Work out the finished part from the listing and answer in its coordinate system (mm). A direction names the side the tool comes from. Give positions to 0.01 mm unless a question says otherwise; leave off trailing zeros. Loops run counter-clockwise (first coordinate to the right, second up) from the corner with the lowest first, then second, coordinate; pieces in that order, holes last.
```python
from build123d import *

# Parameters (mm, degrees)
SKETCH_1_W          = 80.1
SKETCH_1_H          = 60.1
EXTRUDE_1_DEPTH     = 28
CUT_EXTRUDE_1_DEPTH = 108
CUT_EXTRUDE_2_DEPTH = 80
FILLET_1_R          = 2
SKETCH_4_R          = 1.8
CUT_EXTRUDE_3_DEPTH = 80
FILLET_2_R          = 10
FILLET_3_R          = 2


with BuildPart() as part:
    # 草图1 → 凸台-拉伸1 (new body)
    with BuildSketch(Plane.XY):
        with Locations((40.05, -30.05)):
            Rectangle(SKETCH_1_W, SKETCH_1_H)
    extrude(amount=EXTRUDE_1_DEPTH)

    # 草图2 → 切除-拉伸1 (cut)
    with BuildSketch(Plane(origin=(80.1, 0, 0), x_dir=(0, 0, -1), z_dir=(1, 0, 0))):
        with BuildLine():
            ThreePointArc((-4, -32), (-6.928932188, -24.928932188), (-14, -22))
            Line((-14, -22), (-14, -32))
            Line((-14, -32), (-4, -32))
        make_face()
        with BuildLine():
            Line((-14, -32), (-14, -22))
            ThreePointArc((-14, -22), (-21.071067812, -24.928932188), (-24, -32))
            Line((-24, -32), (-14, -32))
        make_face()
        with BuildLine():
            Line((-4, -32), (-14, -32))
            Line((-14, -32), (-14, -42))
            ThreePointArc((-14, -42), (-6.928932188, -39.071067812), (-4, -32))
        make_face()
        with BuildLine():
            Line((-14, -42), (-14, -32))
            Line((-14, -32), (-24, -32))
            ThreePointArc((-24, -32), (-21.071067812, -39.071067812), (-14, -42))
        make_face()
    extrude(amount=-CUT_EXTRUDE_1_DEPTH, mode=Mode.SUBTRACT)

    # 草图3 → 切除-拉伸2 (cut)
    with BuildSketch(Plane(origin=(0, 0, 0), x_dir=(1, 0, 0), z_dir=(0, 1, 0))):
        Polygon((25.05, -11.5), (0, -11.5), (0, -28), (80.1, -28), (80.1, -11.5), (55.05, -11.5), (55.05, -16.5), (25.05, -16.5), align=None)
    extrude(amount=-CUT_EXTRUDE_2_DEPTH, mode=Mode.SUBTRACT)

    # 圆角1
    fillet_1_edges = [part.edges().sort_by_distance(p)[0] for p in [
        (55.05, -50.891229183, 11.5),
        (55.05, -11.158770817, 11.5),
        (25.05, -50.891229183, 11.5),
        (25.05, -11.158770817, 11.5),
        (25.05, -50.891229183, 16.5),
        (25.05, -11.158770817, 16.5),
        (55.05, -50.891229183, 16.5),
        (55.05, -11.158770817, 16.5),
    ]]
    fillet(fillet_1_edges, radius=FILLET_1_R)

    # 草图4 → 切除-拉伸3 (cut)
    with BuildSketch(Plane(origin=(0, 0, 0), x_dir=(-1, 0, 0), z_dir=(0, 0, -1))):
        with Locations((-70.05, -54.5)):
            Circle(SKETCH_4_R)
        with Locations((-10.05, -54.5)):
            Circle(SKETCH_4_R)
        with Locations((-21.05, -3)):
            Circle(SKETCH_4_R)
        with Locations((-59.05, -3)):
            Circle(SKETCH_4_R)
    extrude(amount=-CUT_EXTRUDE_3_DEPTH, mode=Mode.SUBTRACT)

    # 圆角2
    fillet_2_edges = [part.edges().sort_by_distance(p)[0] for p in [
        (0, 0, 5.75),
        (80.1, 0, 5.75),
        (80.1, -60.1, 5.75),
        (0, -60.1, 5.75),
    ]]
    fillet(fillet_2_edges, radius=FILLET_2_R)

    # 圆角3
    # the kernel refuses this fillet: 2 mm, written as the material it takes off along each edge
    with BuildSketch(Plane(origin=(80.1, -10, 0), x_dir=(-1, 0, 0), z_dir=(0, -1, 0)), Plane(origin=(0, -50.1, 0), x_dir=(1, 0, 0), z_dir=(0, 1, 0))) as fillet_3_piece_1:
        with BuildLine():
            CenterArc((FILLET_3_R, -FILLET_3_R), FILLET_3_R, 90, 90)
            Line((0, -FILLET_3_R), (0, 0))
            Line((0, 0), (FILLET_3_R, 0))
        make_face()
    extrude(amount=40.1, mode=Mode.SUBTRACT)
    with BuildSketch(Plane(origin=(10, 0, 0), x_dir=(0, 0, 1), z_dir=(1, 0, 0))) as fillet_3_piece_2:
        with BuildLine():
            CenterArc((FILLET_3_R, FILLET_3_R), FILLET_3_R, 180, 90)
            Line((0, FILLET_3_R), (0, 0))
            Line((0, 0), (FILLET_3_R, 0))
        make_face()
    extrude(amount=60.1, mode=Mode.SUBTRACT)
    with BuildSketch(Plane(origin=(70.1, -60.1, 0), x_dir=(0, 1, 0), z_dir=(-1, 0, 0))) as fillet_3_piece_3:
        with BuildLine():
            CenterArc((FILLET_3_R, -FILLET_3_R), FILLET_3_R, 90, 90)
            Line((0, -FILLET_3_R), (0, 0))
            Line((0, 0), (FILLET_3_R, 0))
        make_face()
    extrude(amount=60.1, mode=Mode.SUBTRACT)
    with BuildSketch(Plane(origin=(10, -10, 0), x_dir=(0, 1, 0), z_dir=(1, 0, 0))) as fillet_3_piece_4:
        with BuildLine():
            CenterArc((10 - FILLET_3_R, FILLET_3_R), FILLET_3_R, 270, 90)
            Line((10, FILLET_3_R), (10, 0))
            Line((10, 0), (10 - FILLET_3_R, 0))
        make_face()
    revolve(axis=Axis((10, -10, 0), (0, 0, 1)), revolution_arc=90, mode=Mode.SUBTRACT)
    with BuildSketch(Plane(origin=(10, -50.1, 0), x_dir=(-1, 0, 0), z_dir=(0, 1, 0))) as fillet_3_piece_5:
        with BuildLine():
            CenterArc((10 - FILLET_3_R, FILLET_3_R), FILLET_3_R, 270, 90)
            Line((10, FILLET_3_R), (10, 0))
            Line((10, 0), (10 - FILLET_3_R, 0))
        make_face()
    revolve(axis=Axis((10, -50.1, 0), (0, 0, 1)), revolution_arc=90, mode=Mode.SUBTRACT)
    with BuildSketch(Plane(origin=(70.1, -10, 0), x_dir=(0, 1, 0), z_dir=(-1, 0, 0))) as fillet_3_piece_6:
        with BuildLine():
            CenterArc((10 - FILLET_3_R, -FILLET_3_R), FILLET_3_R, 0, 90)
            Line((10 - FILLET_3_R, 0), (10, 0))
            Line((10, 0), (10, -FILLET_3_R))
        make_face()
    revolve(axis=Axis((70.1, -10, 0), (0, 0, -1)), revolution_arc=90, mode=Mode.SUBTRACT)
    with BuildSketch(Plane(origin=(70.1, -50.1, 0), x_dir=(1, 0, 0), z_dir=(0, 1, 0))) as fillet_3_piece_7:
        with BuildLine():
            CenterArc((10 - FILLET_3_R, -FILLET_3_R), FILLET_3_R, 0, 90)
            Line((10, -FILLET_3_R), (10, 0))
            Line((10, 0), (10 - FILLET_3_R, 0))
        make_face()
    revolve(axis=Axis((70.1, -50.1, 0), (0, 0, -1)), revolution_arc=90, mode=Mode.SUBTRACT)


solid = part.part
```
Q1. Which of the six approach directions +Z, -Z, +X, -X, +Y, -Y give full straight-line access (tool end or side, diameter ignored) to faces 4 (the face through (69, -51, 11.5)), 5 (the face through (71.85, -54.42, 5.67)), 6 (the face through (12, -51, 11.5))?
Q2. Given pin 1 (0.5 mm diameter, centred on y = -14.5, z = 14, fed in from +X); pin 2 (6 mm diameter, centred on x = 64, z = 4, fed in from +Y); pin 3 (3 mm diameter, centred on x = 59.05, y = -3, fed in from -Z); pin 4 (2 mm diameter, centred on y = -53.5, z = 10.5, fed in from -X), each flat-ended and moving along its own axis, determine where each tip first touches the part or whether it passes through.
Q3. Section B-B on x = 45 is taken. Give the vertices of the cut face in (y, z).
Q4. Section A-A on z = 8 is taken. Give the vertices of the cut face in (x, y), plus the area to 3 significant figures.
Q5. Section D-D on x = 21.05 is taken. Give the vertices of the cut face in (y, z).
Q6. Determine the mould class of faces 1 (the face through (24.45, -51.02, 12.07)), 2 (the face through (60.85, -2.92, 5.67)), 3 (the face through (39.63, -0.6, 0.57)) for opening direction Y: +Y half, -Y half, draft (parallel to the pull), parting line (faces both ways), or undercut.
Q7. Consider line 1 along Y through (x, z) = (21.05, 8.25); line 2 along X through (y, z) = (-3, 3); line 3 along Y through (x, z) = (10.05, 2.5). Determine where each line is inside the solid, lowest interval first.
Q8. Section C-C on z = 3 is taken. Give the vertices of the cut face in (x, y).
Check result:
1. face 4: +Z, +X, +Y, -Y
1. face 5: +Z, -Z
1. face 6: +Z, -X, +Y, -Y
2. pin 1: stops at x = 55.05
2. pin 2: stops at y = 0
2. pin 3: passes through
2. pin 4: stops at x = 0.29
3. outline: (-60.1, 2) arc R2 ccw to (-58.1, 0) - (-2, 0) arc R2 ccw to (0, 2) - (0, 16.5) - (-22.32, 16.5) arc R10 cw (long way) to (-41.68, 16.5) - (-60.1, 16.5) - close
4. outline: (0, -50.1) arc R10 ccw to (10, -60.1) - (70.1, -60.1) arc R10 ccw to (80.1, -50.1) - (80.1, -40) - (0, -40) - close; (0, -24) - (80.1, -24) - (80.1, -10) arc R10 ccw to (70.1, 0) - (10, 0) arc R10 ccw to (0, -10) - close; hole circle Ø3.6 at (10.05, -54.5); hole circle Ø3.6 at (21.05, -3); hole circle Ø3.6 at (59.05, -3); hole circle Ø3.6 at (70.05, -54.5)
4. area: 3,410 mm2
5. outline: (-60.1, 2) arc R2 ccw to (-58.1, 0) - (-4.8, 0) - (-4.8, 11.5) - (-22.32, 11.5) arc R10 cw to (-41.68, 11.5) - (-60.1, 11.5) - close; (-1.2, 0.17) arc R2 ccw to (0, 2) - (0, 11.5) - (-1.2, 11.5) - close
6. face 1: draft
6. face 2: undercut
6. face 3: +Y half
7. line 1: y = -60.1 to -40.18, -23.82 to -4.8, -1.2 to 0
7. line 2: x = 2.86 to 19.25, 22.85 to 57.25, 60.85 to 77.24
7. line 3: y = -60.1 to -56.3, -52.7 to 0
8. outline: (0, -50.1) arc R10 ccw to (10, -60.1) - (70.1, -60.1) arc R10 ccw to (80.1, -50.1) - (80.1, -10) arc R10 ccw to (70.1, 0) - (10, 0) arc R10 ccw to (0, -10) - close; hole circle Ø3.6 at (10.05, -54.5); hole circle Ø3.6 at (21.05, -3); hole circle Ø3.6 at (59.05, -3); hole circle Ø3.6 at (70.05, -54.5)
